Check sheet for the modelled part. Datum: model origin and axes. Units: mm. Face numbers are marked on the shaded views. A direction names the side the tool comes from. Give positions to 0.01 mm unless a question says otherwise; leave off trailing zeros. Write each loop counter-clockwise with the first axis right and the second up, starting at its lowest first coordinate (ties: lowest second). Pieces come first, ordered by that corner, then holes.
from build123d import *

# Parameters (mm, degrees)
SKETCH_R              = 28
SKETCH_R_2            = 7.2
PAD_DEPTH             = 7.5
POCKET_DEPTH          = 166.601597
POLARPATTERN_COUNT    = 3
SKETCH003_R           = 1.7
POCKET001_DEPTH       = 7.501
SKETCH007_R           = 8.6
POCKET005_DEPTH       = 3.5
POCKET006_DEPTH       = 4.3
POLARPATTERN001_COUNT = 3
POCKET007_DEPTH       = 2.3
POLARPATTERN002_COUNT = 3


with BuildPart() as part:
    # Sketch → Pad (new body)
    with BuildSketch(Plane.XY.offset(25)):
        Circle(SKETCH_R)
        Circle(SKETCH_R_2, mode=Mode.SUBTRACT)
    extrude(amount=PAD_DEPTH)

    # Sketch002 → Pocket (cut, through all)
    with BuildSketch(Plane.XY.offset(32.5)):
        with BuildLine():
            ThreePointArc((-4.175823, 11.25), (0, 10.5), (4.175823, 11.25))
            ThreePointArc((8.200179, 8.761111), (6.311893, 10.205881), (4.175823, 11.25))
            ThreePointArc((8.200179, 8.761111), (0, 38.5), (-8.200179, 8.761111))
            ThreePointArc((-4.175823, 11.25), (-6.311893, 10.205881), (-8.200179, 8.761111))
        make_face()
    pocket = extrude(amount=-POCKET_DEPTH, mode=Mode.SUBTRACT)

    # PolarPattern: Pocket ×3 about axis
    polarpattern_axis = Axis((0, 0, 32.5), (0, 0, 1))
    for i in range(1, POLARPATTERN_COUNT):
        add(pocket.rotate(polarpattern_axis, i * 360 / POLARPATTERN_COUNT), mode=Mode.SUBTRACT)

    # Sketch003 → Pocket001 (cut, through all)
    with BuildSketch(Plane.XY.offset(32.5)):
        with Locations((0, 22.5)):
            Circle(SKETCH003_R)
        with Locations((-19.485572, -11.25)):
            Circle(SKETCH003_R)
        with Locations((19.485572, -11.25)):
            Circle(SKETCH003_R)
        with Locations((-19.485572, 11.25)):
            Circle(SKETCH003_R)
        with Locations((19.485572, 11.25)):
            Circle(SKETCH003_R)
        with Locations((0, -22.5)):
            Circle(SKETCH003_R)
    extrude(amount=-POCKET001_DEPTH, mode=Mode.SUBTRACT)

    # Sketch007 → Pocket005 (cut)
    with BuildSketch(Plane.XY.offset(32.5)):
        Circle(SKETCH007_R)
    extrude(amount=-POCKET005_DEPTH, mode=Mode.SUBTRACT)

    # Sketch005 → Pocket006 (cut)
    with BuildSketch(Plane.XY.offset(32.5)):
        with BuildLine():
            Line((-2.35, -8.16869), (-2.35, -18.047645))
            ThreePointArc((-2.35, -18.047645), (0, -18.2), (2.35, -18.047645))
            Line((2.35, -8.16869), (2.35, -18.047645))
            ThreePointArc((-2.35, -8.16869), (0, -8.5), (2.35, -8.16869))
        make_face()
    pocket006 = extrude(amount=-POCKET006_DEPTH, mode=Mode.SUBTRACT)

    # PolarPattern001: Pocket006 ×3 about axis
    polarpattern001_axis = Axis((0, 0, 32.5), (0, 0, 1))
    for i in range(1, POLARPATTERN001_COUNT):
        add(pocket006.rotate(polarpattern001_axis, i * 360 / POLARPATTERN001_COUNT), mode=Mode.SUBTRACT)

    # Sketch009 → Pocket007 (cut)
    with BuildSketch(Plane(origin=(0, 0, 25), x_dir=(1, 0, 0), z_dir=(0, 0, -1))):
        with BuildLine():
            Line((2.35, 12.785832), (2.35, 17.946796))
            ThreePointArc((2.35, 17.946796), (0, 18.1), (-2.35, 17.946796))
            Line((-2.35, 12.785832), (-2.35, 17.946796))
            ThreePointArc((2.35, 12.785832), (0, 13), (-2.35, 12.785832))
        make_face()
    pocket007 = extrude(amount=-POCKET007_DEPTH, mode=Mode.SUBTRACT)

    # PolarPattern002: Pocket007 ×3 about axis
    polarpattern002_axis = Axis((0, 0, 25), (0, 0, -1))
    for i in range(1, POLARPATTERN002_COUNT):
        add(pocket007.rotate(polarpattern002_axis, i * 360 / POLARPATTERN002_COUNT), mode=Mode.SUBTRACT)


solid = part.part
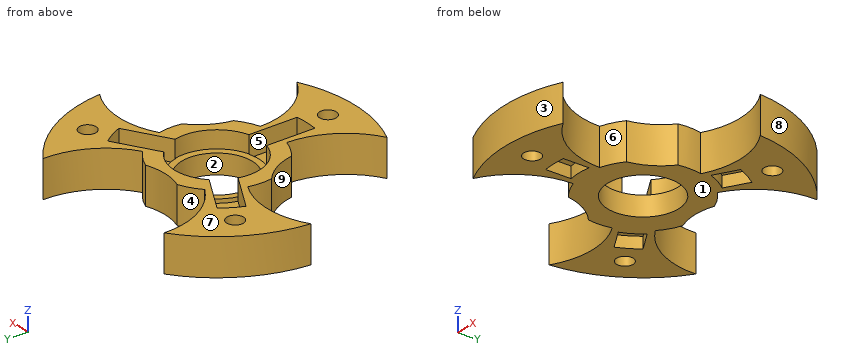
1) Draft check along Y on the marked faces 1, 2, 3 and 4. Enter one of: +Y half, -Y half, draft (parallel to the pull), parting line (faces both ways), or undercut.
2) Sectioned sample at A-A on y = 0. Record the boundary of the cut face in (x, z).
3) Gauge pin test, flat ends, axial feed: pin 1 (3 mm diameter, centred on x = -9, z = 26.5, fed in from +Y); pin 2 (4 mm diameter, centred on x = 22, z = 27, fed in from +Y); pin 3 (1.2 mm diameter, centred on y = -16, z = 26.5, fed in from +X). Record the tip position at first contact, or that the pin passes through.
4) Sectioned sample at B-B on z = 26.5. Give the number of separate pieces and of enclosed holes in the cut face, then the cut area to 3 significant figures.
5) Scan lines: L1, parallel to X at y = -11.5, z = 30; L2, parallel to X at y = 9, z = 29; L3, parallel to Y at x = 10, z = 27.25. Record each from-to range of solid material in increasing order.
6) Access from +Z, -Z, +X, -X, +Y, -Y to the whole of each face (thin tool, end or side, straight path). Record for the marked faces 5, 6, 7, 8 and 9.
7) Sectioned sample at D-D on x = -5. Record the boundary of the cut face in (y, z).
Answers below:
1. face 1: draft
1. face 2: undercut
1. face 3: -Y half
1. face 4: +Y half
2. outline: (-12, 25) - (-7.2, 25) - (-7.2, 29) - (-8.6, 29) - (-8.6, 32.5) - (-12, 32.5) - close; (7.2, 25) - (12, 25) - (12, 32.5) - (8.6, 32.5) - (8.6, 29) - (7.2, 29) - close
3. pin 1: stops at y = 10.43
3. pin 2: stops at y = 19.6
3. pin 3: stops at x = 4.41
4. separate pieces: 1
4. enclosed holes: 7
4. area: 780 mm2
5. L1: x = -3.49 to -2.35, 2.35 to 3.49
5. L2: x = -26.51 to -15.82, -10.89 to -8.59, -7.94 to 7.94, 8.59 to 10.89, 15.82 to 26.51
5. L3: y = -26.15 to -24.14, -3.9 to 8.31, 8.49 to 10.01
6. face 5: +Z
6. face 6: +Z, -Z, +X
6. face 7: +Z, +X, -X, +Y, -Y
6. face 8: +Z, -Z, +X, +Y
6. face 9: +Z, -Z, -X
7. outline: (-27.55, 25) - (-18.04, 25) - (-18.04, 32.5) - (-27.55, 32.5) - close; (-10.91, 25) - (-5.18, 25) - (-5.18, 29) - (-7, 29) - (-7, 32.5) - (-10.91, 32.5) - close; (5.18, 25) - (10.91, 25) - (10.91, 32.5) - (7, 32.5) - (7, 29) - (5.18, 29) - close
